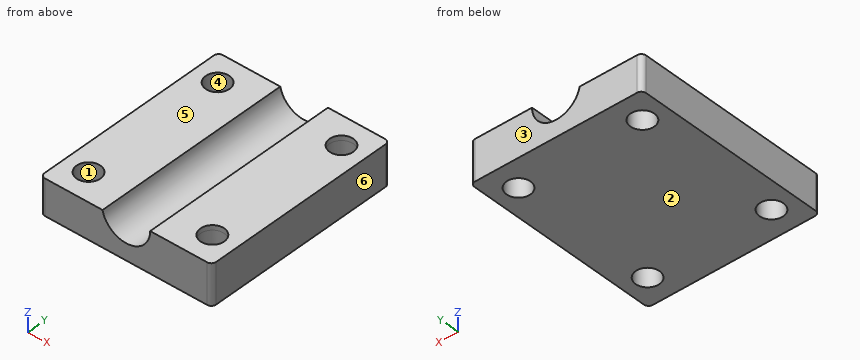
Autodesk Inventor part; units mm, degrees
ref_plane "YZ Plane" through (0, 0, 0) normal (1, 0, 0) x (0, 1, 0)
ref_plane "XZ Plane" through (0, 0, 0) normal (0, 1, 0) x (-1, 0, 0)
ref_plane "XY Plane" through (0, 0, 0) normal (0, 0, 1) x (1, 0, 0)
sketch "Szkic1" plane through (0, 0, 0) normal (0, 0, 1) x (1, 0, 0)
  line L0 (-10.3866, 5.557) -> (25.6134, 5.557)
  line L1 (25.6134, 5.557) -> (25.6134, -36.443)
  line L2 (25.6134, -36.443) -> (-10.3866, -36.443)
  line L3 (-10.3866, -36.443) -> (-10.3866, 5.557)
  point P0 (0, 0)
  point P1 (20.6134, -0.193)
  point P2 (20.6134, -30.693)
  point P3 (-5.3866, -0.193)
  point P4 (-5.3866, -30.693)
  dimension "d0" = 36
  dimension "d1" = 42
  dimension "d2" = 5
  dimension "d3" = 5
  dimension "d4" = 5
  dimension "d5" = 5
  dimension "d6" = 5.75
  dimension "d7" = 5.75
  dimension "d8" = 5.75
  dimension "d9" = 5.75
extrude "Wyciągnięcie proste1" add sketch "Szkic1" along normal blind 7.5
hole "Otwór1" at (20.6134, -0.193, 0) at (20.6134, -30.693, 0) at (-5.3866, -0.193, 0) at (-5.3866, -30.693, 0) direction (0, 0, 1) diameter 5 end through all
sketch "Szkic2" plane through (-10.3866, -36.443, 0) normal (0, -1, 0) x (1, 0, 0)
  line L0 (36, 0) -> (0, 0)
  line L1 (36, 0) -> (36, 7.5)
  line L2 (0, 7.5) -> (36, 7.5)
  line L3 (0, 0) -> (0, 7.5)
  line L4 (36, 7.5) -> (0, 7.5)
  circle A0 centre (18, 8.5) radius 5.05
  point P0 (10.3866, 0)
  dimension "d19" = 36
  dimension "d25" = 8.5
  dimension "d26" = 18
  dimension "d27" = 10.1
extrude "Wyciągnięcie proste2" cut sketch "Szkic2" against normal through all contours A0 L2 | L2 A0
fillet "Zaokrąglenie1" radius 1 4 edges at (-10.3866, -36.443, 3.75) (-10.3866, 5.557, 3.75) (25.6134, -36.443, 3.75) (25.6134, 5.557, 3.75)
sketch "Szkic3" plane through (0, 0, 7.5) normal (0, 0, 1) x (1, 0, 0)
  arc A0 (25.6134, 4.557) -> (24.6134, 5.557) centre (24.6134, 4.557) ccw
  line L0 (24.6134, 5.557) -> (12.5634, 5.557)
  line L1 (12.5634, 5.557) -> (12.5634, -36.443)
  line L2 (12.5634, -36.443) -> (24.6134, -36.443)
  arc A1 (24.6134, -36.443) -> (25.6134, -35.443) centre (24.6134, -35.443) ccw
  line L3 (25.6134, -35.443) -> (25.6134, 4.557)
  circle A2 centre (20.6134, -0.193) radius 2.5
  circle A3 centre (20.6134, -30.693) radius 2.5
  point P0 (0, 0)
extrude "Wyciągnięcie proste3" add sketch "Szkic3" along normal blind 1
sketch "Szkic4" plane through (-9.3866, -36.443, 0) normal (0, -1, 0) x (1, 0, 0)
  line L0 (34, 8.5) -> (34, 0)
  line L1 (21.95, 8.5) -> (34, 8.5)
  line L2 (21.95, 7.5) -> (21.95, 8.5)
  arc A0 (12.05, 7.5) -> (21.95, 7.5) centre (17, 8.5) ccw
  line L3 (0, 7.5) -> (12.05, 7.5)
  line L4 (0, 0) -> (0, 7.5)
  line L5 (34, 0) -> (0, 0)
  circle A1 centre (17, 8.5) radius 5.05
  point P0 (9.3866, 0)
  dimension "d30" = 10.1
extrude "Wyciągnięcie proste4" cut sketch "Szkic4" against normal through all contours A1 L2 L1 | L1 L2 A0 A1
properties part number "3DP_ABS_X_Axis_Linear_Shaft_Clamp_Bottom"
Design review of the part built by this model. Coordinates are the model's own, in mm. Face numbers are marked on the shaded views. A direction names the side the tool comes from. Round coordinates to 2 decimals unless told otherwise and drop trailing zeros. Loops run counter-clockwise (first coordinate to the right, second up) from the corner with the lowest first, then second, coordinate; pieces in that order, holes last. Notation, with made-up numbers: M 72,63 L 130,63 A21 ccw 130,98 Z; hole C 44,-32 d7. An arc over 180 degrees is marked long. Answer as a JSON object with one key per item and string values.
Item 1: We need section C-C on z = 1.75. Give the boundary of the cut face in (x, y), and give its area (3 significant figures).
Answer sheet:
{"outline": "M -10.39,-35.44 A1 ccw -9.39,-36.44 L 24.61,-36.44 A1 ccw 25.61,-35.44 L 25.61,4.56 A1 ccw 24.61,5.56 L -9.39,5.56 A1 ccw -10.39,4.56 Z; hole C -5.39,-30.69 d5; hole C -5.39,-0.19 d5; hole C 20.61,-30.69 d5; hole C 20.61,-0.19 d5", "area": "1,430 mm^2"}
Item 2: The part is to be moulded in two halves that separate along Y. For the marked faces 1, 2, 3 and 4, say which applies: pulls with the +Y half, pulls with the -Y half, needs draft (parallel to the pull), parting line crosses it, or undercut.
Answer sheet:
{"face 1": "undercut", "face 2": "needs draft", "face 3": "pulls with the +Y half", "face 4": "undercut"}
Item 3: We need section B-B on x = 22. Give the boundary of the cut face in (y, z), and give its area (3 significant figures).
Answer sheet:
{"outline": "M -36.44,0 L -32.77,0 L -32.77,8.5 L -36.44,8.5 Z; M -28.61,0 L -2.27,0 L -2.27,8.5 L -28.61,8.5 Z; M 1.89,0 L 5.56,0 L 5.56,8.5 L 1.89,8.5 Z", "area": "286 mm^2"}
Item 4: Machinability: for the marked faces 5 and 6, which of the approach directions +Z, -Z, +X, -X, +Y, -Y give a long, thin tool a straight path to every point of the face, cutting with its end or side? Answer none if there is none.
Answer sheet:
{"face 5": "+Z, -X, +Y, -Y", "face 6": "+Z, -Z, +X, +Y, -Y"}
Item 5: We need section A-A on z = 5.5. Give the boundary of the cut face in (x, y).
Answer sheet:
{"outline": "M -10.39,-35.44 A1 ccw -9.39,-36.44 L 3.55,-36.44 L 3.55,5.56 L -9.39,5.56 A1 ccw -10.39,4.56 Z; M 11.68,-36.44 L 24.61,-36.44 A1 ccw 25.61,-35.44 L 25.61,4.56 A1 ccw 24.61,5.56 L 11.68,5.56 Z; hole C -5.39,-30.69 d5; hole C -5.39,-0.19 d5; hole C 20.61,-30.69 d5; hole C 20.61,-0.19 d5"}
Item 6: We need section D-D on y = -26. Give the boundary of the cut face in (x, z).
Answer sheet:
{"outline": "M -10.39,0 L 25.61,0 L 25.61,8.5 L 12.66,8.5 A5.05 cw 2.66,7.5 L -10.39,7.5 Z"}
Item 7: Wall thickness on L1, parallel to Y at x = 20.5, z = 1.75; L2, parallel to Y at x = 22.5, z = 3.75; L3, parallel to X at y = 2, z = 5.5: over which ranges is each line inside the solid? List them lowest first. Write a range as from..to.
Answer sheet:
{"L1": "y = -36.44..-33.19, -28.2..-2.69, 2.3..5.56", "L2": "y = -36.44..-32.33, -29.05..-1.83, 1.45..5.56", "L3": "x = -10.39..-6.59, -4.19..3.55, 11.68..19.41, 21.81..25.61"}
Item 8: Clearance check with a flat-ended pin moving along its axis: P1, Ø12, axis at x = -1, y = -19, coming from the +Z side. State where the tip first meets the part, or that it passes through.
Answer sheet:
{"P1": "stops at z = 7.5"}
